```python
from build123d import *

# Parameters (mm, degrees)
BASE_DEPTH            = 3
WALLS_DEPTH           = 17.8
PEDESTAL_DEPTH        = 3.6
SKETCH8_R             = 1.3
THRUHOLE_DEPTH        = 7.6
NUT_HOLE_DEPTH        = 2.4
MIRROR2_COPY_1_DEPTH  = 3.6
SKETCH6_R             = 3.05
EYELET_DEPTH          = 3
SKETCH4_W             = 11
SKETCH4_H             = 7
HOLE_USB_PORT_DEPTH   = 2.6
SKETCH5_W             = 8.5
SKETCH5_H             = 6
HOLE_SCREW_TERM_DEPTH = 2.6
CIRPATTERN1_COUNT     = 2
CHAMFER1_SIZE         = 0.4


with BuildPart() as part:
    # Sketch1 → base (new body)
    with BuildSketch(Plane(origin=(0, 0, 0), x_dir=(1, 0, 0), z_dir=(0, 1, 0))):
        with BuildLine():
            Line((-23.46, 13.6), (23.46, 13.6))
            ThreePointArc((23.46, 13.6), (26.387422074, 12.387422074), (27.6, 9.46))
            Line((27.6, 9.46), (27.6, -9.46))
            ThreePointArc((27.6, -9.46), (26.387422074, -12.387422074), (23.46, -13.6))
            Line((23.46, -13.6), (-23.46, -13.6))
            ThreePointArc((-23.46, -13.6), (-26.387422074, -12.387422074), (-27.6, -9.46))
            Line((-27.6, -9.46), (-27.6, 9.46))
            ThreePointArc((-27.6, 9.46), (-26.387422074, 12.387422074), (-23.46, 13.6))
        make_face()
    extrude(amount=-BASE_DEPTH)

    # Sketch1_3 → walls (add)
    with BuildSketch(Plane(origin=(0, 0, 0), x_dir=(1, 0, 0), z_dir=(0, 1, 0))):
        with BuildLine():
            ThreePointArc((-27.6, 9.46), (-26.387422074, 12.387422074), (-23.46, 13.6))
            Line((-23.46, 13.6), (23.46, 13.6))
            ThreePointArc((23.46, 13.6), (26.387422074, 12.387422074), (27.6, 9.46))
            Line((27.6, 9.46), (27.6, -9.46))
            ThreePointArc((27.6, -9.46), (26.387422074, -12.387422074), (23.46, -13.6))
            Line((23.46, -13.6), (-23.46, -13.6))
            ThreePointArc((-23.46, -13.6), (-26.387422074, -12.387422074), (-27.6, -9.46))
            Line((-27.6, -9.46), (-27.6, 9.46))
        make_face()
        with BuildLine():
            Line((-23.46, 12), (23.46, 12))
            ThreePointArc((23.46, 12), (25.256051224, 11.256051224), (26, 9.46))
            Line((26, 9.46), (26, -9.46))
            ThreePointArc((26, -9.46), (25.256051224, -11.256051224), (23.46, -12))
            Line((23.46, -12), (-23.46, -12))
            ThreePointArc((-23.46, -12), (-25.256051224, -11.256051224), (-26, -9.46))
            Line((-26, -9.46), (-26, 9.46))
            ThreePointArc((-26, 9.46), (-25.256051224, 11.256051224), (-23.46, 12))
        make_face(mode=Mode.SUBTRACT)
    extrude(amount=WALLS_DEPTH)

    # Sketch2 → pedestal (add)
    with BuildSketch(Plane(origin=(0, 0, 0), x_dir=(1, 0, 0), z_dir=(0, 1, 0))):
        with BuildLine():
            Line((-26, 6.46), (-23, 6.46))
            ThreePointArc((-23, 6.46), (-21.203948776, 7.203948776), (-20.46, 9))
            Line((-20.46, 9), (-20.46, 12))
            Line((-20.46, 12), (-26, 12))
            Line((-26, 12), (-26, 6.46))
        make_face()
    pedestal = extrude(amount=PEDESTAL_DEPTH)

    # Sketch8 → thruhole (cut, through all)
    with BuildSketch(Plane(origin=(0, 3.6, 0), x_dir=(1, 0, 0), z_dir=(0, 1, 0))):
        with Locations((-22.86, 8.89)):
            Circle(SKETCH8_R)
    thruhole = extrude(amount=-THRUHOLE_DEPTH, mode=Mode.SUBTRACT)

    # Sketch10 → nut hole (cut)
    with BuildSketch(Plane.XZ.offset(3)):
        Polygon((-25.8622214, -8.89), (-24.3611107, -11.49), (-21.3588893, -11.49), (-19.8577786, -8.89), (-21.3588893, -6.29), (-24.3611107, -6.29), align=None)
    nut_hole = extrude(amount=-NUT_HOLE_DEPTH, mode=Mode.SUBTRACT)

    # Mirror1: pedestal across plane
    add(pedestal.mirror(Plane(origin=(0, 0, 0), x_dir=(0, 0, 1), z_dir=(1, 0, 0))))

    # Mirror2: pedestal across plane
    add(pedestal.mirror(Plane.XY))

    # Mirror2 copy 1 sketch → Mirror2 copy 1 (add)
    with BuildSketch(Plane(origin=(0, 0, 0), x_dir=(-1, 0, 0), z_dir=(0, 1, 0))):
        with BuildLine():
            Line((-26, 6.46), (-23, 6.46))
            ThreePointArc((-23, 6.46), (-21.203948776, 7.203948776), (-20.46, 9))
            Line((-20.46, 9), (-20.46, 12))
            Line((-20.46, 12), (-26, 12))
            Line((-26, 12), (-26, 6.46))
        make_face()
    extrude(amount=MIRROR2_COPY_1_DEPTH)

    # Sketch6 → eyelet (add)
    with BuildSketch(Plane(origin=(0, -3, 0), x_dir=(1, 0, 0), z_dir=(0, 1, 0))):
        with BuildLine():
            Line((-18.5, 19.6), (-18.5, 13.6))
            Line((-18.5, 13.6), (-6.5, 13.6))
            Line((-6.5, 13.6), (-6.5, 19.6))
            ThreePointArc((-6.5, 19.6), (-12.5, 25.6), (-18.5, 19.6))
        make_face()
        with Locations((-12.5, 19.6)):
            Circle(SKETCH6_R, mode=Mode.SUBTRACT)
    eyelet = extrude(amount=EYELET_DEPTH)

    # Mirror3: eyelet across plane
    add(eyelet.mirror(Plane(origin=(0, 0, 0), x_dir=(0, 0, 1), z_dir=(1, 0, 0))))

    # Sketch4 → hole_USB_port (cut, through all)
    with BuildSketch(Plane(origin=(-26, 0, 0), x_dir=(0, 0, -1), z_dir=(1, 0, 0))):
        with Locations((0, 6.44)):
            Rectangle(SKETCH4_W, SKETCH4_H)
    extrude(amount=-HOLE_USB_PORT_DEPTH, mode=Mode.SUBTRACT)

    # Sketch5 → hole_screw_term (cut, through all)
    with BuildSketch(Plane.ZY.offset(-26)):
        with Locations((-2.53, 7.6)):
            Rectangle(SKETCH5_W, SKETCH5_H)
    extrude(amount=-HOLE_SCREW_TERM_DEPTH, mode=Mode.SUBTRACT)

    # CirPattern1: thruhole, nut hole ×2 about axis
    cirpattern1_axis = Axis((0, 0, 0), (0, 1, 0))
    for i in range(1, CIRPATTERN1_COUNT):
        add(thruhole.rotate(cirpattern1_axis, i * 360 / CIRPATTERN1_COUNT), mode=Mode.SUBTRACT)
        add(nut_hole.rotate(cirpattern1_axis, i * 360 / CIRPATTERN1_COUNT), mode=Mode.SUBTRACT)

    # Chamfer1
    chamfer1_edges = [part.edges().sort_by_distance(p)[0] for p in [
        (26.387422074, -3, -12.387422074),
        (27.6, -3, 0),
        (0, -3, -13.6),
        (-12.5, 0, -25.6),
        (-18.5, 0, -16.6),
        (-6.5, 0, -16.6),
        (-15.55, -3, -19.6),
        (-12.5, -3, -25.6),
        (-18.5, -3, -16.6),
        (-6.5, -3, -16.6),
        (-15.55, 0, -19.6),
        (12.5, 0, -25.6),
        (6.5, 0, -16.6),
        (18.5, 0, -16.6),
        (15.55, 0, -19.6),
        (12.5, -3, -25.6),
        (18.5, -3, -16.6),
        (6.5, -3, -16.6),
        (15.55, -3, -19.6),
        (26.387422074, -3, 12.387422074),
        (24.16, 3.6, 8.89),
        (25.11166605, -3, 7.59),
        (25.11166605, -3, 10.19),
        (22.86, -3, 11.49),
        (20.60833395, -3, 10.19),
        (20.60833395, -3, 7.59),
        (22.86, -3, 6.29),
        (0, -3, 13.6),
        (-26.387422074, -3, 12.387422074),
        (-27.6, -3, 0),
        (-26.387422074, -3, -12.387422074),
        (-24.16, 3.6, -8.89),
        (-25.11166605, -3, -7.59),
        (-25.11166605, -3, -10.19),
        (-22.86, -3, -11.49),
        (-20.60833395, -3, -10.19),
        (-20.60833395, -3, -7.59),
        (-22.86, -3, -6.29),
    ]]
    chamfer(chamfer1_edges, length=CHAMFER1_SIZE)


solid = part.part
```
Source: CAD feature listing. Evaluate the final solid. Frame: model axes, mm. A direction names the side the tool comes from. Round coordinates to 2 decimals unless told otherwise and drop trailing zeros. Loops run counter-clockwise (first coordinate to the right, second up) from the corner with the lowest first, then second, coordinate; pieces in that order, holes last. Notation, with made-up numbers: M 45,32.25 L 83,32.25 A20 cw 83,40.25 Z; hole C 65.5,1 d8. An arc over 180 degrees is marked long. Use a Markdown table: item, result. Add a question column.
1. Cut plane B-B, the plane x = 12.5. Output: boundary loops of the cut face in (y, z), and give its area (3 significant figures).
2. Cut plane A-A, the plane z = -3. Output: boundary loops of the cut face in (x, y).
3. Pull-direction query (Z, two-part tool) for faces 1 (the flat face through (0, 7, 13.6)), 2 (the flat face through (23, 3.6, -9)), 3 (the flat face through (27.6, 7, 2)); classes: +Z half, -Z half, draft (parallel to the pull), parting line (faces both ways), or undercut.
4. Set-up query: faces 4 (the cylindrical face through (25.236, 10.601, -11.276)), 5 (the flat face through (25.122, -1.614, 10.172)), 6 (the flat face through (-18.5, -2, -17)), 7 (the conical face through (26.211, -2.892, 12.151)). Return all of +Z, -Z, +X, -X, +Y, -Y with unobstructed straight access to the full face (end or side cutting, diameter ignored); none if empty.
5. Ray query, line 1 along X through (y, z) = (0.9, -8.89); line 2 along Z through (x, y) = (22.86, 1.25); line 3 along X through (y, z) = (-1.6, -19.6). Return the intervals inside material, ascending. Write a range as [from, to].
6. Cut plane C-C, the plane z = 4. Output: boundary loops of the cut face in (x, y).
7. Cut plane D-D, the plane x = 0. Output: boundary loops of the cut face in (y, z).
8. Contact query for flat-ended pins moving along their axis: pin 1 (1.3 mm diameter, centred on x = 27, y = 7, fed in from -Z); pin 2 (2.5 mm diameter, centred on y = -1.5, z = -16, fed in from +X); pin 3 (2 mm diameter, centred on x = 23, y = -2, fed in from -Z); pin 4 (10 mm diameter, centred on x = -1, z = -21.5, fed in from -Y). Output: stop coordinate, or through.
Solution:
| question | item | result |
|---|---|---|
| 1 | outline | M -3,-25.2 L -2.6,-25.6 L -0.4,-25.6 L 0,-25.2 L 0,-23.05 L -0.4,-22.65 L -2.6,-22.65 L -3,-23.05 Z; M -3,-16.15 L -2.6,-16.55 L -0.4,-16.55 L 0,-16.15 L 0,-13.6 L 17.8,-13.6 L 17.8,-12 L 0,-12 L 0,12 L 17.8,12 L 17.8,13.6 L -2.6,13.6 L -3,13.2 Z |
| 1 | area | 156 mm2 |
| 2 | outline | M -27.6,-2.6 L -27.2,-3 L 27.2,-3 L 27.6,-2.6 L 27.6,4.6 L 26,4.6 L 26,0 L -26,0 L -26,2.94 L -27.6,2.94 Z; M -27.6,9.94 L -26,9.94 L -26,17.8 L -27.6,17.8 Z; M 26,10.6 L 27.6,10.6 L 27.6,17.8 L 26,17.8 Z |
| 3 | face 1 | +Z half |
| 3 | face 2 | undercut |
| 3 | face 3 | draft |
| 4 | face 4 | +Y |
| 4 | face 5 | -Y |
| 4 | face 6 | -Z, -X, +Y, -Y |
| 4 | face 7 | +Z, +X, -Y |
| 5 | line 1 | x = [-27.6, -24.16], [-21.56, -20.46], [20.46, 27.6] |
| 5 | line 2 | z = [-13.6, -6.46], [6.46, 7.59], [10.19, 13.6] |
| 5 | line 3 | x = [-18.5, -15.55], [-9.45, -6.5], [6.5, 9.45], [15.55, 18.5] |
| 6 | outline | M -27.6,-2.6 L -27.2,-3 L 27.2,-3 L 27.6,-2.6 L 27.6,17.8 L 26,17.8 L 26,0 L -26,0 L -26,2.94 L -27.6,2.94 Z; M -27.6,9.94 L -26,9.94 L -26,17.8 L -27.6,17.8 Z |
| 7 | outline | M -3,-13.2 L -2.6,-13.6 L 17.8,-13.6 L 17.8,-12 L 0,-12 L 0,12 L 17.8,12 L 17.8,13.6 L -2.6,13.6 L -3,13.2 Z |
| 8 | pin 1 | stops at z = -12.42 |
| 8 | pin 2 | stops at x = 18.5 |
| 8 | pin 3 | stops at z = -13.6 |
| 8 | pin 4 | passes through |
